Geometry check sheet. Reference: the model listing, model coordinates, mm. A direction names the side the tool comes from. Coordinates: 2 decimals unless noted, no trailing zeros. Write each loop counter-clockwise with the first axis right and the second up, starting at its lowest first coordinate (ties: lowest second). Pieces come first, ordered by that corner, then holes. Notation, with made-up numbers: (43.5, 12) -> (47.5, 12) arc R25 cw to (47.5, 44) -> close; hole circle Ø7 at (46, 57). An arc over 180 degrees is marked (long way). One line per question, with ' | ' between items.
```python
from build123d import *

# Parameters (mm, degrees)
F1_DEPTH = 15
F3_DEPTH = 13.3


with BuildPart() as f1:
    # F0 (on Top) → F1 (new body)
    with BuildSketch(Plane.XY):
        with BuildLine():
            Line((6.65, 0), (1.65, 0))
            ThreePointArc((1.65, 0), (0, -1.65), (-1.65, 0))
            Line((-1.65, 0), (-6.65, 0))
            ThreePointArc((-6.65, 0), (0, -6.65), (6.65, 0))
        make_face()
        with BuildLine():
            ThreePointArc((-1.65, 0), (0, 1.65), (1.65, 0))
            Line((1.65, 0), (6.65, 0))
            ThreePointArc((6.65, 0), (0, 6.65), (-6.65, 0))
            Line((-6.65, 0), (-1.65, 0))
        make_face()
        with BuildLine():
            Line((6.65, -11.65), (6.65, 0))
            ThreePointArc((6.65, 0), (0, -6.65), (-6.65, 0))
            Line((-6.65, 0), (-6.65, -11.65))
            Line((-6.65, -11.65), (6.65, -11.65))
        make_face()
    extrude(amount=F1_DEPTH)

    # F2 (on face) → F3 (cut, through all)
    with BuildSketch(Plane.YZ.offset(6.65)):
        with BuildLine():
            ThreePointArc((-1.7433336736, 6.75), (-1.6921187257, 7.1234467199), (-1.675, 7.5))
            ThreePointArc((-1.675, 7.5), (-1.6921187257, 7.8765532801), (-1.7433336736, 8.25))
            Line((-1.7433336736, 8.25), (-1.7433336736, 6.75))
        make_face()
        with BuildLine():
            ThreePointArc((-1.7433336736, 8.25), (-1.6921187257, 7.8765532801), (-1.675, 7.5))
            ThreePointArc((-1.675, 7.5), (-1.6921187257, 7.1234467199), (-1.7433336736, 6.75))
            Line((-1.7433336736, 6.75), (9.3667274341, 6.75))
            Line((9.3667274341, 6.75), (9.3667274341, 8.25))
            Line((9.3667274341, 8.25), (-1.7433336736, 8.25))
        make_face()
        with BuildLine():
            Line((-1.7433336736, 6.75), (-1.7433336736, 8.25))
            ThreePointArc((-1.7433336736, 8.25), (-9.975, 7.5), (-1.7433336736, 6.75))
        make_face()
    extrude(amount=-F3_DEPTH, mode=Mode.SUBTRACT)


solid = f1.part
```
(1) Tool access check on faces 4 (the face through (0, 2, 6.75)), 5 (the face through (0.15, 6.65, 3.33)). Record the directions out of +Z, -Z, +X, -X, +Y, -Y that give a thin tool (end or side, any length) a straight path to the whole face; none if there is none.
Answers below:
face 4: +X, -X, +Y | face 5: +Z, -Z, +Y
(2) Cross-section at D-D (y = 0.5). Record the cut outline in (x, z).
Answers below:
outline: (-6.63, 0) -> (-1.57, 0) -> (-1.57, 6.75) -> (-6.63, 6.75) -> close; (-6.63, 8.25) -> (-1.57, 8.25) -> (-1.57, 15) -> (-6.63, 15) -> close; (1.57, 0) -> (6.63, 0) -> (6.63, 6.75) -> (1.57, 6.75) -> close; (1.57, 8.25) -> (6.63, 8.25) -> (6.63, 15) -> (1.57, 15) -> close
(3) Material ranges on line 1 (Z direction, x = 4.25, y = 0.75); line 2 (Y direction, x = 0, z = 5.75); line 3 (Y direction, x = 0, z = 12.75), recorded low to high.
Answers below:
line 1: z = 0 to 6.75, 8.25 to 15 | line 2: y = -11.65 to -9.59, -2.06 to -1.65, 1.65 to 6.65 | line 3: y = -11.65 to -1.65, 1.65 to 6.65
(4) Depth check by flat-ended pin: P1, Ø2, axis at x = 0, y = 0, coming from the -Z side; P2, Ø6.5, axis at x = 1, y = 1, coming from the -Z side; P3, Ø1, axis at x = -3.5, z = 3, coming from the +Y side; P4, Ø3, axis at y = 2.5, z = 9.5, coming from the +X side. Enter the tip coordinate at first touch or a pass-through.
Answers below:
P1: passes through | P2: stops at z = 0 | P3: stops at y = 5.93 | P4: stops at x = 6.57
(5) Cross-section at C-C (z = 12.25). Record the cut outline in (x, y).
Answers below:
outline: (-6.65, -11.65) -> (6.65, -11.65) -> (6.65, 0) arc R6.65 ccw to (-6.65, 0) -> close; hole circle Ø3.3 at (0, 0)
(6) Draft check along Z on faces 1 (the face through (0.15, 6.65, 11.58)), 2 (the face through (0, -2, 0)), 3 (the face through (0, 3, 8.25)). Enter one of: pulls with the +Z half, pulls with the -Z half, needs draft (parallel to the pull), parting line crosses it, or undercut.
Answers below:
face 1: needs draft | face 2: pulls with the -Z half | face 3: undercut
(7) Cross-section at B-B (y = 4.5). Record the cut outline in (x, z).
Answers below:
outline: (-4.9, 0) -> (4.9, 0) -> (4.9, 6.75) -> (-4.9, 6.75) -> close; (-4.9, 8.25) -> (4.9, 8.25) -> (4.9, 15) -> (-4.9, 15) -> close
(8) Cross-section at A-A (z = 4.75). Record the cut outline in (x, y).
Answers below:
outline: (-6.65, -11.65) -> (6.65, -11.65) -> (6.65, -8.93) -> (-6.65, -8.93) -> close; (-6.65, -2.72) -> (6.65, -2.72) -> (6.65, 0) arc R6.65 ccw to (-6.65, 0) -> close; hole circle Ø3.3 at (0, 0)
